Source: CAD feature listing. Evaluate the final solid. Frame: model axes, mm. A direction names the side the tool comes from. Give positions to 0.01 mm unless a question says otherwise; leave off trailing zeros. Write each loop counter-clockwise with the first axis right and the second up, starting at its lowest first coordinate (ties: lowest second). Pieces come first, ordered by that corner, then holes. Notation, with made-up numbers: M 3,-34.5 L 25,-34.5 A19 ccw 25,-29.5 Z; hole C 36,37 d9. An arc over 180 degrees is marked long. Answer as a JSON object with one key per item and string values. Group by question number.
```python
from build123d import *

# Parameters (mm, degrees)
SKETCH1_R           = 13
BOSS_EXTRUDE1_DEPTH = 1.5
SKETCH2_R           = 6.5
BOSS_EXTRUDE2_DEPTH = 6
SKETCH3_R           = 3
CUT_EXTRUDE1_DEPTH  = 6
SKETCH4_R           = 1.25
CUT_EXTRUDE5_DEPTH  = 8
SKETCH6_R           = 1
CUT_EXTRUDE6_DEPTH  = 6
SKETCH7_R           = 12
SKETCH7_R_2         = 2
BOSS_EXTRUDE3_DEPTH = 1.5
SKETCH8_R           = 6.5
SKETCH8_R_2         = 2
BOSS_EXTRUDE4_DEPTH = 0.8
CUT_EXTRUDE8_START  = -10.8
SKETCH9_R           = 1.25
CUT_EXTRUDE8_DEPTH  = 10.8
CUT_EXTRUDE9_START  = -10.8
SKETCH10_R          = 2
CUT_EXTRUDE9_DEPTH  = 10.8
CUT_EXTRUDE10_DEPTH = 0.8
CHAMFER4_SIZE       = 1


with BuildPart() as part:
    # Sketch1 → Boss-Extrude1 (new body)
    with BuildSketch(Plane(origin=(0, 0, 0), x_dir=(1, 0, 0), z_dir=(0, 1, 0))):
        with Locations(Location((0, 0, 0), (0, 0, 270))):
            Circle(SKETCH1_R)
    extrude(amount=BOSS_EXTRUDE1_DEPTH)

    # Sketch2 → Boss-Extrude2 (add)
    with BuildSketch(Plane(origin=(0, 1.5, 0), x_dir=(1, 0, 0), z_dir=(0, 1, 0))):
        with Locations(Location((0, 0, 0), (0, 0, 270))):
            Circle(SKETCH2_R)
    extrude(amount=BOSS_EXTRUDE2_DEPTH)

    # Sketch3 → Cut-Extrude1 (cut)
    with BuildSketch(Plane(origin=(0, 7.5, 0), x_dir=(1, 0, 0), z_dir=(0, 1, 0))):
        with Locations(Location((0, 0, 0), (0, 0, 270))):
            Circle(SKETCH3_R)
    extrude(amount=-CUT_EXTRUDE1_DEPTH, mode=Mode.SUBTRACT)

    # Sketch4 → Cut-Extrude5 (cut, symmetric)
    with BuildSketch(Plane.XZ):
        with Locations(Location((-8.5, 0, 0), (0, 0, 90))):
            Circle(SKETCH4_R)
        with Locations(Location((0, 8.5, 0), (0, 0, 90))):
            Circle(SKETCH4_R)
        with Locations(Location((8.5, 0, 0), (0, 0, 90))):
            Circle(SKETCH4_R)
        with Locations(Location((0, -8.5, 0), (0, 0, 90))):
            Circle(SKETCH4_R)
    extrude(amount=CUT_EXTRUDE5_DEPTH, both=True, mode=Mode.SUBTRACT)

    # Sketch6 → Cut-Extrude6 (cut)
    with BuildSketch(Plane(origin=(0, 7.5, 0), x_dir=(1, 0, 0), z_dir=(0, 1, 0))):
        with Locations(Location((0, 4.75, 0), (0, 0, 270))):
            Circle(SKETCH6_R)
        with Locations(Location((0, -4.75, 0), (0, 0, 270))):
            Circle(SKETCH6_R)
    extrude(amount=-CUT_EXTRUDE6_DEPTH, mode=Mode.SUBTRACT)

    # Sketch7 → Boss-Extrude3 (add)
    with BuildSketch(Plane.XZ):
        with Locations(Location((0, 0, 0), (0, 0, 270))):
            Circle(SKETCH7_R)
        with Locations(Location((0, 0, 0), (0, 0, 270))):
            Circle(SKETCH7_R_2, mode=Mode.SUBTRACT)
    extrude(amount=BOSS_EXTRUDE3_DEPTH)

    # Sketch8 → Boss-Extrude4 (add)
    with BuildSketch(Plane.XZ.offset(1.5)):
        with Locations(Location((0, 0, 0), (0, 0, 90))):
            Circle(SKETCH8_R)
        with Locations(Location((0, 0, 0), (0, 0, 270))):
            Circle(SKETCH8_R_2, mode=Mode.SUBTRACT)
    extrude(amount=BOSS_EXTRUDE4_DEPTH)

    # Sketch9 → Cut-Extrude8 (cut)
    with BuildSketch(Plane(origin=(0, 0, 0), x_dir=(1, 0, 0), z_dir=(0, 1, 0)).offset(CUT_EXTRUDE8_START)):
        with Locations(Location((8.5, 0, 0), (0, 0, 90))):
            Circle(SKETCH9_R)
        with Locations(Location((0, -8.5, 0), (0, 0, 90))):
            Circle(SKETCH9_R)
        with Locations(Location((-8.5, 0, 0), (0, 0, 90))):
            Circle(SKETCH9_R)
        with Locations(Location((0, 8.5, 0), (0, 0, 90))):
            Circle(SKETCH9_R)
    extrude(amount=CUT_EXTRUDE8_DEPTH, mode=Mode.SUBTRACT)

    # Sketch10 → Cut-Extrude9 (cut)
    with BuildSketch(Plane.XZ.offset(CUT_EXTRUDE9_START)):
        with Locations(Location((0, 0, 0), (0, 0, 90))):
            Circle(SKETCH10_R)
    extrude(amount=CUT_EXTRUDE9_DEPTH, mode=Mode.SUBTRACT)

    # Sketch11 → Cut-Extrude10 (cut)
    with BuildSketch(Plane.XZ.offset(2.3)):
        with BuildLine():
            Line((-6.109126461, 2.220039164), (-3.889087297, 0))
            Line((-3.889087297, 0), (0, 3.889087297))
            Line((0, 3.889087297), (-2.220039164, 6.109126461))
            ThreePointArc((-2.220039164, 6.109126461), (-4.596194078, 4.596194078), (-6.109126461, 2.220039164))
        make_face()
    extrude(amount=-CUT_EXTRUDE10_DEPTH, mode=Mode.SUBTRACT)

    # Chamfer4
    chamfer4_edges = [part.edges().sort_by_distance(p)[0] for p in [
        (0, 1.5, -2),
    ]]
    chamfer(chamfer4_edges, length=CHAMFER4_SIZE - 0.0001)  # a hair under: the kernel refuses the full size


solid = part.part
```
(1) Ray query, L1, parallel to X at y = 0.5, z = 0; L2, parallel to X at y = -0.35, z = 0; L3, parallel to X at y = 4.95, z = 0. Return the intervals inside material, ascending. Write a range as [from, to].
(2) Section B-B, the plane y = -1. Return loops of the section in (x, z).
(3) Contact query for flat-ended pins moving along their axis: pin 1 Ø2 at (x, z) = (0, -8.5) entering from -Y; pin 2 Ø3 at (x, y) = (-6.5, 5) entering from +Z; pin 3 Ø4 at (x, y) = (-5.5, 5) entering from +Z; pin 4 Ø5 at (x, y) = (-6, 0) entering from +Z. Output: stop coordinate, or through.
(4) Section A-A, the plane x = 8.5. Return loops of the section in (y, z), plus the area to 3 significant figures.
(5) Section C-C, the plane z = -8.5. Return loops of the section in (x, y).
(6) Pull-direction query (Z, two-part tool) for faces 1 (the flat face through (-3, 7.5, 1)), 2 (the cylindrical face through (4.419, -1.894, -4.767)), 3 (the cylindrical face through (0.9, 4.54, 2.86)); classes: pulls with the +Z half, pulls with the -Z half, needs draft (parallel to the pull), parting line crosses it, or undercut.
(7) Access query for faces 4 (the flat face through (-1.09, -1.91, 4.98)), 5 (the flat face through (-2, -1.5, 3)), 6 (the cylindrical face through (-0.61, 4.54, -5.54)). Directions: +Z, -Z, +X, -X, +Y, -Y. A direction counts if a zero-diameter tool reaches every point of the face in a straight line with its end or side. Return the directions, or none.
(8) Section D-D, the plane y = 2.75. Return loops of the section in (x, z), plus the area to 3 significant figures.
Reported:
{
 "1": {"L1": "x = [-13, -9.75], [-7.25, -2], [2, 7.25], [9.75, 13]", "L2": "x = [-12, -9.75], [-7.25, -2], [2, 7.25], [9.75, 12]", "L3": "x = [-6.5, -3], [3, 6.5]"},
 "2": {"outline": "C 0,0 d24; hole C -8.5,0 d2.5; hole C 0,0 d4; hole C 0,-8.5 d2.5; hole C 0,8.5 d2.5; hole C 8.5,0 d2.5"},
 "3": {"pin 1": "passes through", "pin 2": "stops at z = 4.15", "pin 3": "stops at z = 5.48", "pin 4": "stops at z = 12.52"},
 "4": {"outline": "M -1.5,-8.47 L 0,-8.47 L 0,-9.84 L 1.5,-9.84 L 1.5,-1.25 L -1.5,-1.25 Z; M -1.5,1.25 L 1.5,1.25 L 1.5,9.84 L 0,9.84 L 0,8.47 L -1.5,8.47 Z", "area": "47.4 mm2"},
 "5": {"outline": "M -9.84,0 L -8.47,0 L -8.47,-1.5 L -1.25,-1.5 L -1.25,1.5 L -9.84,1.5 Z; M 1.25,-1.5 L 8.47,-1.5 L 8.47,0 L 9.84,0 L 9.84,1.5 L 1.25,1.5 Z"},
 "6": {"face 1": "needs draft", "face 2": "parting line crosses it", "face 3": "undercut"},
 "7": {"face 4": "-X, -Y", "face 5": "-Y", "face 6": "+Y"},
 "8": {"outline": "C 0,0 d13; hole C 0,0 d6; hole C 0,-4.75 d2; hole C 0,4.75 d2", "area": "98.2 mm2"}
}
